```python
from build123d import *


with BuildPart() as part:
    # Sketch2 → Revolve2 (revolve)
    with BuildSketch(Plane(origin=(0, 0, 0), x_dir=(0, 0, -1), z_dir=(1, 0, 0)), mode=Mode.PRIVATE) as revolve2_sk:
        Polygon((-0.9, 19.5), (0.9, 19.5), (1.15, 18.6), (1.15, 18.3), (0.9, 18.3), (0.9, 17.757735027), (1, 17.7), (0.9, 17.642264973), (0.9, 17.5), (-0.9, 17.5), (-0.9, 17.642264973), (-1, 17.7), (-0.9, 17.757735027), (-0.9, 18.3), (-1.15, 18.3), (-1.15, 18.6), align=None)
    revolve(revolve2_sk.sketch.rotate(Axis((0, 0, 0), (0, 0, -1)), 90), axis=Axis((0, 0, 0), (0, 0, -1)))


solid = part.part
```
Verification items for the finished model (mm, model axes). A direction names the side the tool comes from. Give positions to 0.01 mm unless a question says otherwise; leave off trailing zeros. Order: outer loops, then holes, each group sorted by start corner. A loop starts at its lowest first (then second) coordinate and runs counter-clockwise, first axis right, second up. Notation, with made-up numbers: (-1.75, 31.25) -> (19.25, 31.25) arc R34 cw to (19.25, 61.25) -> close; hole circle Ø8 at (24, 27.25). An arc over 180 degrees is marked (long way). Use a Markdown table: item, result.
1) Depth check by flat-ended pin: pin 1 Ø3 at (x, y) = (7.5, -12) entering from +Z; pin 2 Ø1 at (y, z) = (6.5, -1) entering from -X; pin 3 Ø1 at (y, z) = (-7.5, 0) entering from -X. Enter the tip coordinate at first touch or a pass-through.
Results:
| item | result |
|---|---|
| pin 1 | through |
| pin 2 | x = -18.55 |
| pin 3 | x = -18.2 |
2) Mould release check, pull along Y, two halves, no side actions. Record for faces 3 (the flat face through (-15, -10, -0.9)), 4 (the cylindrical face through (-2.539, -19.334, -0.013)): pulls with the +Y half, pulls with the -Y half, needs draft (parallel to the pull), parting line crosses it, or undercut.
Results:
| item | result |
|---|---|
| face 3 | undercut |
| face 4 | parting line crosses it |
3) Tool access check on faces 1 (the flat face through (15, -10, 0.9)), 2 (the cylindrical face through (-3.794, 17.084, 0.013)). Record the directions out of +Z, -Z, +X, -X, +Y, -Y that give a thin tool (end or side, any length) a straight path to the whole face; none if there is none.
Results:
| item | result |
|---|---|
| face 1 | +Z |
| face 2 | +Z, -Z |
4) Material ranges on probe 1 along X at (y, z) = (-0.5, -0.25); probe 2 along Y at (x, z) = (0, -0.1); probe 3 along Y at (x, z) = (-13.5, 0.2), recorded low to high.
Results:
| item | result |
|---|---|
| probe 1 | -19.49 to -17.49, 17.49 to 19.49 |
| probe 2 | -19.5 to -17.5, 17.5 to 19.5 |
| probe 3 | -14.07 to -11.14, 11.14 to 14.07 |
5) Section check C-C, the plane z = 0. Record the boundary of the cut face in (x, y).
Results:
| item | result |
|---|---|
| outline | circle Ø39 at (0, 0); hole circle Ø35 at (0, 0) |
